Answer from the drawing. Dimensions are ordinates in mm from the lowest x, y and z of the part. Round coordinates to 2 decimals unless told otherwise and drop trailing zeros. Loops run counter-clockwise (first coordinate to the right, second up) from the corner with the lowest first, then second, coordinate; pieces in that order, holes last.
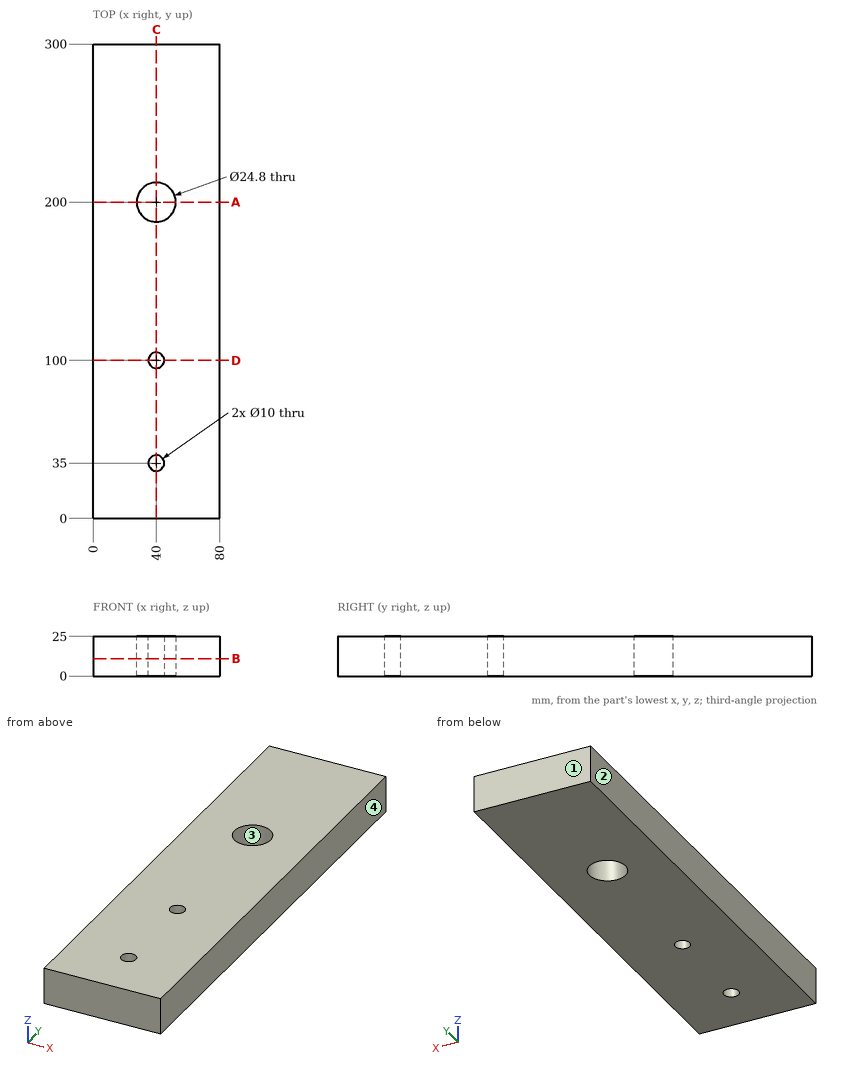
1. Determine the mould class of the marked faces 1, 2, 3 and 4 for opening direction X: +X half, -X half, draft (parallel to the pull), parting line (faces both ways), or undercut.
Answer key:
face 1: draft
face 2: -X half
face 3: undercut
face 4: +X half
2. Find section C-C (x = 40). Write down the section's boundary in (y, z).
Answer key:
outline: (0, 0) - (30, 0) - (30, 25) - (0, 25) - close; (40, 0) - (95, 0) - (95, 25) - (40, 25) - close; (105, 0) - (187.6, 0) - (187.6, 25) - (105, 25) - close; (212.4, 0) - (300, 0) - (300, 25) - (212.4, 25) - close
3. Find section D-D (y = 100). Write down the section's boundary in (x, z).
Answer key:
outline: (0, 0) - (35, 0) - (35, 25) - (0, 25) - close; (45, 0) - (80, 0) - (80, 25) - (45, 25) - close
4. Find section B-B (z = 11). Write down the section's boundary in (x, y).
Answer key:
outline: (0, 0) - (80, 0) - (80, 300) - (0, 300) - close; hole circle Ø24.8 at (40, 200); hole circle Ø10 at (40, 35); hole circle Ø10 at (40, 100)
5. Consider probe 1 along Y at (x, z) = (40, 17.75); probe 2 along Y at (x, z) = (30, 7.75); probe 3 along Y at (x, z) = (46.5, 6). Determine where each line is inside the solid, lowest interval first.
Answer key:
probe 1: y = 0 to 30, 40 to 95, 105 to 187.6, 212.4 to 300
probe 2: y = 0 to 192.67, 207.33 to 300
probe 3: y = 0 to 189.44, 210.56 to 300
6. Given pin 1 (5 mm diameter, centred on x = 26.5, y = 96, fed in from -Z); pin 2 (8 mm diameter, centred on x = 40, y = 100, fed in from -Z), each flat-ended and moving along its own axis, determine where each tip first touches the part or whether it passes through.
Answer key:
pin 1: stops at z = 0
pin 2: passes through
7. Find section A-A (y = 200). Write down the section's boundary in (x, z).
Answer key:
outline: (0, 0) - (27.6, 0) - (27.6, 25) - (0, 25) - close; (52.4, 0) - (80, 0) - (80, 25) - (52.4, 25) - close
